Autodesk Inventor part; units mm, degrees
ref_plane "YZ Plane" through (0, 0, 0) normal (1, 0, 0) x (0, 1, 0)
ref_plane "XZ Plane" through (0, 0, 0) normal (0, 1, 0) x (-1, 0, 0)
ref_plane "XY Plane" through (0, 0, 0) normal (0, 0, 1) x (1, 0, 0)
sketch "스케치1" plane through (0, 0, 0) normal (0, 1, 0) x (-1, 0, 0)
  line L0 (10, 22.5) -> (-10, 22.5)
  line L1 (-10, 22.5) -> (-10, -22.5)
  line L2 (-10, -22.5) -> (10, -22.5)
  line L3 (10, -22.5) -> (10, 22.5)
  line L4 (10, 22.5) -> (-10, -22.5) construction
  line L5 (-10, 22.5) -> (10, -22.5) construction
  line L6 (-7.5, 20) -> (-7.5, -20) construction
  line L7 (0, 13.5) -> (0, -13.5) construction
  circle A0 centre (0, 13.5) radius 8
  circle A1 centre (0, -13.5) radius 8
  line L8 (7.5, 20) -> (7.5, -20) construction
  circle A2 centre (-7.5, 20) radius 1
  circle A3 centre (7.5, -20) radius 1
  point P0 (0, 0)
  point P1 (0, 0)
  dimension "d0" = 20
  dimension "d1" = 45
  dimension "d2" = 27
  dimension "d3" = 40
  dimension "d4" = 20
  dimension "d5" = 10
  dimension "d6" = 9
  dimension "d7" = 16
  dimension "d8" = 16
  dimension "d9" = 40
  dimension "d10" = 20
  dimension "d11" = 15
  dimension "d12" = 7.5
  dimension "d13" = 2
  dimension "d14" = 2
extrude "돌출1" add sketch "스케치1" along normal blind 1.2 contours L3 L2 L1 L0 | A0 | A1
sketch "스케치2" plane through (0, 1.2, 0) normal (0, 1, 0) x (1, 0, 0)
  line L0 (0, -13.5) -> (0, 13.5)
  line L1 (-10, 22.5) -> (-10, -22.5)
  line L2 (10, -22.5) -> (10, 22.5)
  circle A0 centre (0, -13.5) radius 8
  circle A1 centre (0, 13.5) radius 8
  point P0 (0, 0)
  point P1 (-10, 0)
  dimension "d17" = 27
  dimension "d20" = 10
  dimension "d21" = 13.5
  dimension "d22" = 16
  dimension "d23" = 16
extrude "돌출2" add sketch "스케치2" along normal blind 13.8
properties part number "초음파센서"
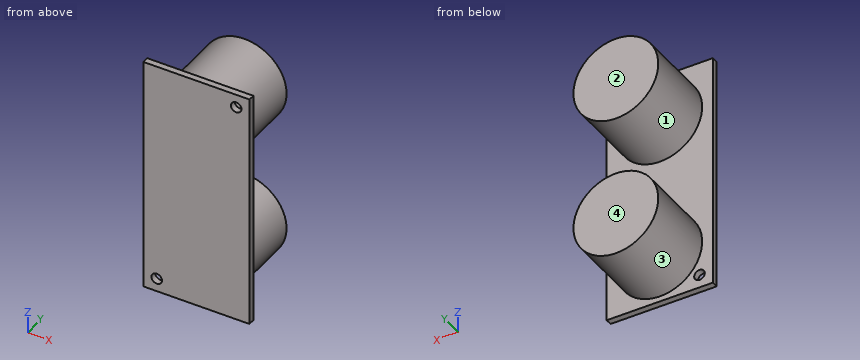
For this review, take the finished solid that the model builds, in its own axes (mm). Face numbers are marked on the shaded views. A direction names the side the tool comes from. Give positions to 0.01 mm unless a question says otherwise; leave off trailing zeros. Order: outer loops, then holes, each group sorted by start corner. A loop starts at its lowest first (then second) coordinate and runs counter-clockwise, first axis right, second up.
1) Wall thickness on line 1 (Z direction, x = -7.5, y = 0.7); line 2 (Z direction, x = 7.5, y = 0.6); line 3 (Y direction, x = 4.75, z = 0): over which ranges is each line inside the solid? List them lowest first.
2) Take a section at A-A (y = 5.5). Give the boundary of the cut face in (x, z), then the cut area to 3 significant figures.
3) Take a section at D-D (z = 13.5). Give the boundary of the cut face in (x, y).
4) For the marked faces 1 and 2, list the 3-axis set-ups (+Z, -Z, +X, -X, +Y, -Y) from which the entire face can be reached by the end or side of a thin tool; tool diameter is ignored.
5) The part is to be moulded in two halves that separate along Z. For the marked faces 3 and 4, say which applies: released by +Z, released by -Z, zero draft, split by the parting line, or undercut.
6) Insertion check: pin 1 (1 mm diameter, centred on y = 6.5, z = 13.5, fed in from +X); pin 2 (4 mm diameter, centred on x = 6, z = -4.5, fed in from +Y); pin 3 (6 mm diameter, centred on x = 7.5, y = 6, fed in from +Z). Each pin has a flat end and moves straight along its axis. Give the tip position at first contact, or say it passes through.
7) Take a section at C-C (x = -7.5). Give the boundary of the cut face in (y, z).
8) Take a section at B-B (z = 19.5). Give the boundary of the cut face in (x, y).
Derived:
1. line 1: z = -22.5 to -21, -19 to 22.5
1. line 2: z = -22.5 to 19, 21 to 22.5
1. line 3: y = 0 to 1.2
2. outline: circle Ø16 at (0, -13.5); circle Ø16 at (0, 13.5)
2. area: 402 mm2
3. outline: (-10, 0) - (10, 0) - (10, 1.2) - (8, 1.2) - (8, 15) - (-8, 15) - (-8, 1.2) - (-10, 1.2) - close
4. face 1: +Y
4. face 2: +Z, -Z, +X, -X, +Y
5. face 3: undercut
5. face 4: zero draft
6. pin 1: stops at x = 8
6. pin 2: stops at y = 1.2
6. pin 3: stops at z = 20.11
7. outline: (0, -22.5) - (1.2, -22.5) - (1.2, -21) - (0, -21) - close; (0, -19) - (1.2, -19) - (1.2, -16.28) - (15, -16.28) - (15, -10.72) - (1.2, -10.72) - (1.2, 10.72) - (15, 10.72) - (15, 16.28) - (1.2, 16.28) - (1.2, 22.5) - (0, 22.5) - close
8. outline: (-10, 0) - (6.63, 0) - (6.63, 1.2) - (5.29, 1.2) - (5.29, 15) - (-5.29, 15) - (-5.29, 1.2) - (-10, 1.2) - close; (8.37, 0) - (10, 0) - (10, 1.2) - (8.37, 1.2) - close
